The listing builds one solid part. Answer for the finished solid, in the listing's coordinates (mm). A direction names the side the tool comes from. Give positions to 0.01 mm unless a question says otherwise; leave off trailing zeros. Order: outer loops, then holes, each group sorted by start corner. A loop starts at its lowest first (then second) coordinate and runs counter-clockwise, first axis right, second up.
```python
from build123d import *

# Parameters (mm, degrees)
SKIZZE1_W                       = 100
SKIZZE1_H                       = 100
AUFSATZ_LINEAR_AUSTRAGEN1_DEPTH = 10
SCHNITT_LINEAR_AUSTRAGEN1_DEPTH = 5


with BuildPart() as part:
    # Skizze1 → Aufsatz-Linear austragen1 (new body)
    with BuildSketch(Plane(origin=(0, 0, 0), x_dir=(1, 0, 0), z_dir=(0, 1, 0))):
        Rectangle(SKIZZE1_W, SKIZZE1_H)
    extrude(amount=AUFSATZ_LINEAR_AUSTRAGEN1_DEPTH)

    # Skizze3 → Schnitt-Linear austragen1 (cut)
    with BuildSketch(Plane(origin=(0, 0, 0), x_dir=(1, 0, 0), z_dir=(0, 1, 0))):
        with BuildLine():
            Line((50, 31.52163249), (-35.561044575, 31.52163249))
            Line((-35.561044575, 31.52163249), (-35.561044575, -22.426016782))
            Line((-35.561044575, -22.426016782), (-7.198956111, -22.426016782))
            Line((-7.198956111, -22.426016782), (-7.198956111, -50))
            ThreePointArc((-7.198956111, -50), (2.801043889, -60), (12.801043889, -50))
            Line((12.801043889, -50), (12.801043889, -2.426016782))
            Line((12.801043889, -2.426016782), (-15.561044575, -2.426016782))
            Line((-15.561044575, -2.426016782), (-15.561044575, 11.52163249))
            Line((-15.561044575, 11.52163249), (50, 11.52163249))
            ThreePointArc((50, 11.52163249), (60, 21.52163249), (50, 31.52163249))
        make_face()
    extrude(amount=SCHNITT_LINEAR_AUSTRAGEN1_DEPTH, mode=Mode.SUBTRACT)


solid = part.part
```
1) Find section C-C (z = 43). Write down the section's boundary in (x, y).
Geometry says:
outline: (-50, 0) - (-7.2, 0) - (-7.2, 5) - (12.8, 5) - (12.8, 0) - (50, 0) - (50, 10) - (-50, 10) - close
2) Find section B-B (x = -10.5). Write down the section's boundary in (y, z), then the cut area to 3 significant figures.
Geometry says:
outline: (0, -50) - (10, -50) - (10, 50) - (0, 50) - (0, 22.43) - (5, 22.43) - (5, 2.43) - (0, 2.43) - (0, -11.52) - (5, -11.52) - (5, -31.52) - (0, -31.52) - close
area: 800 mm2
3) Find section D-D (x = -30). Write down the section's boundary in (y, z).
Geometry says:
outline: (0, -50) - (10, -50) - (10, 50) - (0, 50) - (0, 22.43) - (5, 22.43) - (5, -31.52) - (0, -31.52) - close
4) Straight lines are drawn through the part: probe 1 along Z at (x, y) = (14.5, 3.75); probe 2 along X at (y, z) = (3.5, 25.5); probe 3 along X at (y, z) = (0.5, -30). For each, find the intervals that lie inside material, in ascending order.
Geometry says:
probe 1: z = -50 to -31.52, -11.52 to 50
probe 2: x = -50 to -7.2, 12.8 to 50
probe 3: x = -50 to -35.56
5) For a pull along X with two mould halves and no side action, classify faces 1 (the flat face through (-50, 5, 1)), 2 (the flat face through (-12, 0, -34)), 3 (the flat face through (-7.199, 2, 36)) as +X half, -X half, draft (parallel to the pull), parting line (faces both ways), or undercut.
Geometry says:
face 1: -X half
face 2: draft
face 3: undercut
6) A tool of negligible diameter and unlimited length cuts with its end or side. For faces 4 (the flat face through (12.801, 2, 27)), 5 (the flat face through (-1, 6, 50)), 6 (the flat face through (-35.561, 2, -5)), 7 (the flat face through (17, 2, -11.522)), from which of +Z, -Z, +X, -X, +Y, -Y can it reach the whole face along a straight path? Write none if from no direction.
Geometry says:
face 4: +Z, -Y
face 5: +Z, +X, -X, +Y, -Y
face 6: -Y
face 7: +X, -Y
7) Given P1, Ø2, axis at y = 3.5, z = -14.5, coming from the +X side; P2, Ø1.5, axis at x = 10.5, y = 1.5, coming from the +Z side, each flat-ended and moving along its own axis, determine where each tip first touches the part or whether it passes through.
Geometry says:
P1: stops at x = -35.56
P2: stops at z = 2.43
8) Find section A-A (y = 3.25). Write down the section's boundary in (x, z), then the cut area to 3 significant figures.
Geometry says:
outline: (-50, -50) - (50, -50) - (50, -31.52) - (-35.56, -31.52) - (-35.56, 22.43) - (-7.2, 22.43) - (-7.2, 50) - (-50, 50) - close; (-15.56, -11.52) - (50, -11.52) - (50, 50) - (12.8, 50) - (12.8, 2.43) - (-15.56, 2.43) - close
area: 6,490 mm2
